Geometry: see drawing. Coordinates: mm, zero at the bounding-box minimum. A direction names the side the tool comes from. Give positions to 0.01 mm unless a question says otherwise; leave off trailing zeros. Write each loop counter-clockwise with the first axis right and the second up, starting at its lowest first coordinate (ties: lowest second). Pieces come first, ordered by that corner, then holes.
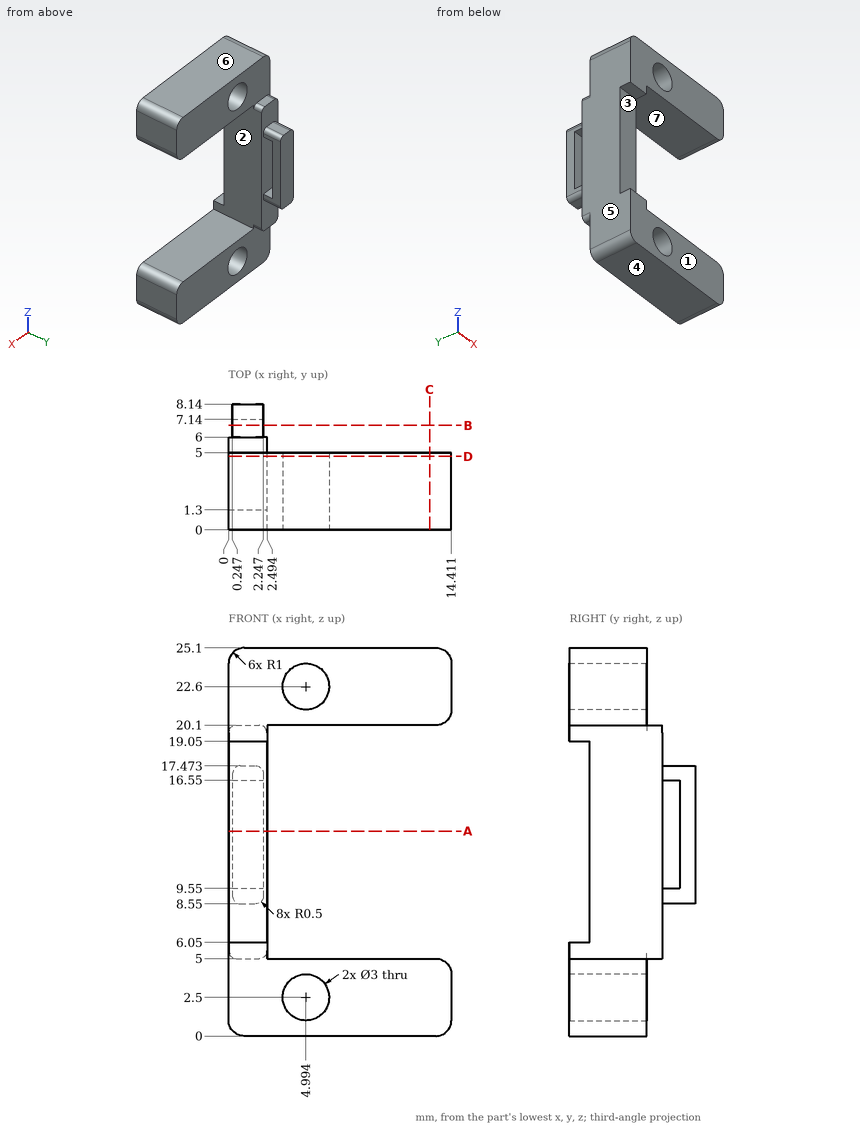
Q1. Section C-C, the plane x = 13. Return the cut outline in (y, z).
Q2. Section A-A, the plane z = 13.25. Return the cut outline in (x, y) (1 decimal).
Q3. Section B-B, the plane y = 6.75. Return the cut outline in (x, z).
Q4. Material intervals for line 1 along X through (y, z) = (3.4, 22.6) (1 decimal); line 2 along Z through (x, y) = (5.5, 3.75); line 3 along Z through (x, y) = (12, 2.25), sorted ascending.
Q5. Access query for the marked faces 1, 2 and 3. Directions: +Z, -Z, +X, -X, +Y, -Y. A direction counts if a zero-diameter tool reaches every point of the face in a straight line with its end or side. Return the directions, or none.
Q6. Mould query, pull axis Z, two halves, no side actions, for the marked faces 4, 5, 6 and 7. Classes: +Z half, -Z half, draft (parallel to the pull), parting line (faces both ways), or undercut.
Q7. Section D-D, the plane y = 4.75. Return the cut outline in (x, z) (1 decimal).
Q8. Pin query (flat end, axial travel): pin 1 (4 mm diameter, centred on x = 8.5, z = 21, fed in from +Y); pin 2 (0.9 mm diameter, centred on x = 1, y = 7, fed in from -Z); pin 3 (1.1 mm diameter, centred on y = 6.5, z = 11.5, fed in from +X); pin 4 (2.5 mm diameter, centred on x = 4.99, z = 2.5, fed in from +Y). Return the tip coordinate at first contact, or that it passes through.
Solutions:
1. outline: (0, 0) - (5, 0) - (5, 5) - (0, 5) - close; (0, 20.1) - (5, 20.1) - (5, 25.1) - (0, 25.1) - close
2. outline: (0, 1.3) - (2.5, 1.3) - (2.5, 6) - (0, 6) - close; (0.2, 7.1) - (2.2, 7.1) - (2.2, 8.1) - (0.2, 8.1) - close
3. outline: (0.25, 9.05) arc R0.5 ccw to (0.75, 8.55) - (1.75, 8.55) arc R0.5 ccw to (2.25, 9.05) - (2.25, 9.55) - (0.25, 9.55) - close; (0.25, 16.55) - (2.25, 16.55) - (2.25, 16.97) arc R0.5 ccw to (1.75, 17.47) - (0.75, 17.47) arc R0.5 ccw to (0.25, 16.97) - close
4. line 1: x = 0 to 3.5, 6.5 to 14.4
4. line 2: z = 0 to 1.09, 3.91 to 5, 20.1 to 21.19, 24.01 to 25.1
4. line 3: z = 0 to 5, 20.1 to 25.1
5. face 1: +Z, -Z, +X, -X, -Y
5. face 2: +X, +Y, -Y
5. face 3: +X, -X, -Y
6. face 4: -Z half
6. face 5: draft
6. face 6: +Z half
6. face 7: undercut
7. outline: (0, 1) arc R1 ccw to (1, 0) - (13.4, 0) arc R1 ccw to (14.4, 1) - (14.4, 4) arc R1 ccw to (13.4, 5) - (2.5, 5) - (2.5, 20.1) - (13.4, 20.1) arc R1 ccw to (14.4, 21.1) - (14.4, 24.1) arc R1 ccw to (13.4, 25.1) - (1, 25.1) arc R1 ccw to (0, 24.1) - close; hole circle Ø3 at (5, 2.5); hole circle Ø3 at (5, 22.6)
8. pin 1: stops at y = 5
8. pin 2: stops at z = 8.55
8. pin 3: stops at x = 2.49
8. pin 4: passes through
